Study the drawing (mm; zero at the part's minimum x, y, z) and answer. A direction names the side the tool comes from. Coordinates: 2 decimals unless noted, no trailing zeros. Write each loop counter-clockwise with the first axis right and the second up, starting at its lowest first coordinate (ties: lowest second). Pieces come first, ordered by that corner, then holes. Notation, with made-up numbers: M 68.25,-22.5 L 82.25,-22.5 A21 cw 82.25,7.5 Z; hole C -5.75,33 d7. An arc over 180 degrees is marked long. Answer as CSV lines item,"result". Start each with the question number.
(1) Find the intervals of material crossed by L1, parallel to Y at x = 23, z = 7; L2, parallel to Z at x = 37, y = 101; L3, parallel to Y at x = 56, z = 4, in increasing order. Write a range as [from, to].
(2) A cutting plane is placed at A-A on z = 7.5. Give the vertices of the cut face in (x, y).
(3) A cutting plane is placed at D-D on z = 21. Give the vertices of the cut face in (x, y).
(4) A cutting plane is placed at C-C on x = 10. Give the vertices of the cut face in (y, z), then the cut area to 3 significant figures.
(5) Flat-ended cylindrical pins translate along their axes: P1, Ø6, axis at x = 19, y = 104, coming from the +Z side; P2, Ø16, axis at x = 32, z = 21.5, coming from the -Y side. Find the tip coordinate at first contact, or state that the pin passes through.
(6) For the marked faces 1 and 2, determine the directions among +Z, -Z, +X, -X, +Y, -Y from which every point of the face is accessible in a straight line to the end or side of a thin tool.
(7) A cutting plane is placed at B-B on y = 15. Give the vertices of the cut face in (x, z).
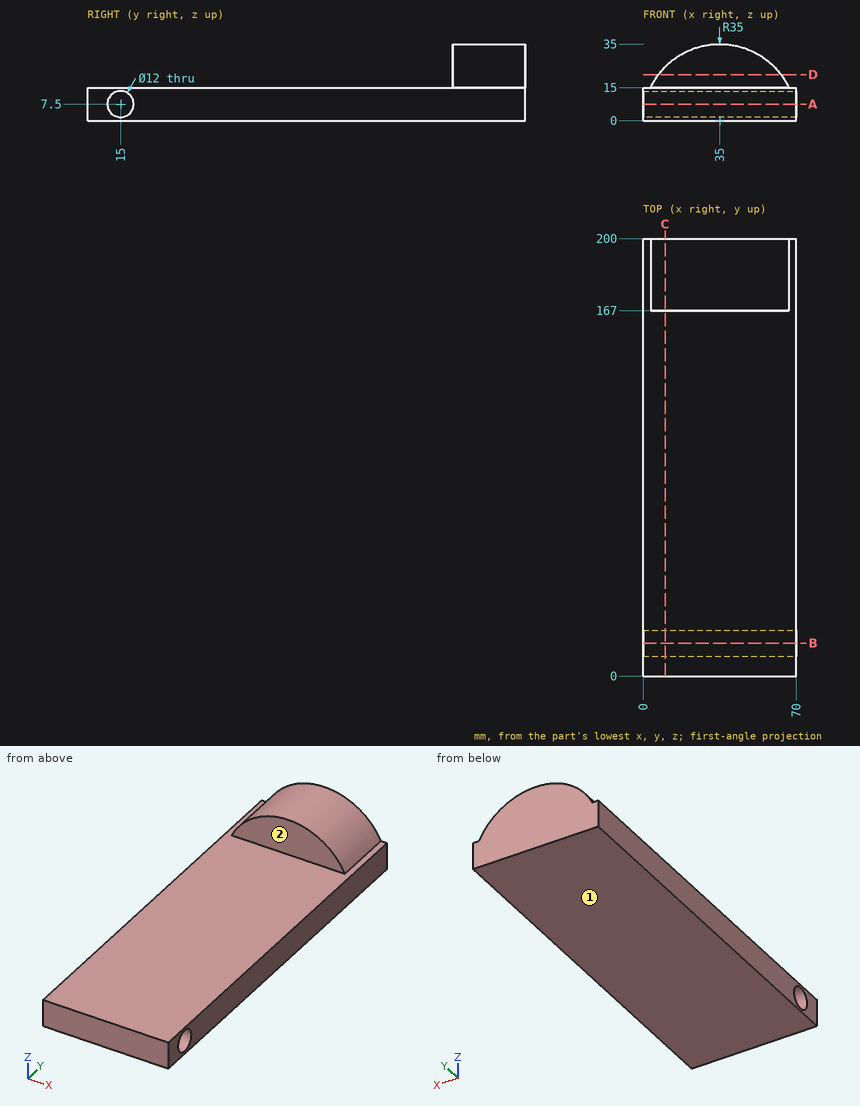
Here are the results:
1,L1,"y = [0, 9.02], [20.98, 200]"
1,L2,"z = [0, 15]"
1,L3,"y = [0, 10.13], [19.87, 200]"
2,outline,"M 0,0 L 70,0 L 70,9 L 0,9 Z; M 0,21 L 70,21 L 70,200 L 0,200 Z"
3,outline,"M 7,167 L 63,167 L 63,200 L 7,200 Z"
4,outline,"M 0,0 L 200,0 L 200,24.49 L 167,24.49 L 167,15 L 0,15 Z; hole C 15,7.5 d12"
4,area,"3,200 mm^2"
5,P1,"stops at z = 15"
5,P2,"stops at y = 0"
6,face 1,"-Z, +X, -X, +Y, -Y"
6,face 2,"+Z, +X, -X, -Y"
7,outline,"M 0,0 L 70,0 L 70,1.5 L 0,1.5 Z; M 0,13.5 L 70,13.5 L 70,15 L 0,15 Z"
